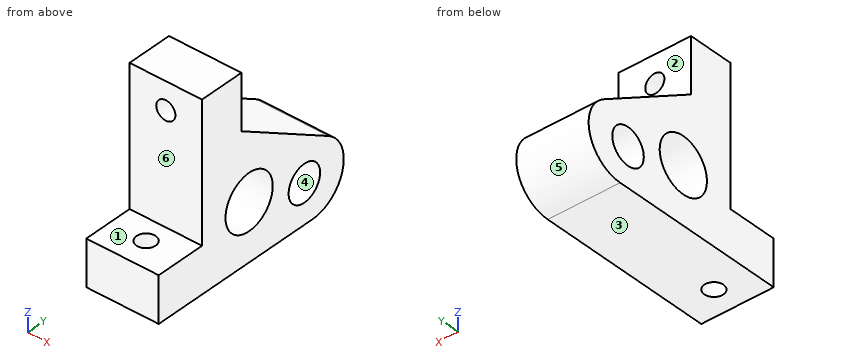
```python
from build123d import *

# Parameters (mm, degrees)
RESSALTO_EXTRUS_O1_DEPTH                       = 7.94
BROCA_DE_ROSQUEAR_PARA_TARRAXA_DE_M5X0_8_D     = 4.2
BROCA_DE_ROSQUEAR_PARA_TARRAXA_DE_M5X0_8_DEPTH = 20
BROCA_DE_ROSQUEAR_PARA_TARRAXA_DE_M5X0_8_TIP   = 1.2618073
BROCA_DE_ROSQUEAR_PARA_TARRAXA_DE_M5_2_D       = 4.2
BROCA_DE_ROSQUEAR_PARA_TARRAXA_DE_M5_2_DEPTH   = 20
BROCA_DE_ROSQUEAR_PARA_TARRAXA_DE_M5_2_TIP     = 1.2618073
BROCA_DE_ROSQUEAR_PARA_TARRAXA_DE_M5_3_D       = 4.2
BROCA_DE_ROSQUEAR_PARA_TARRAXA_DE_M5_3_DEPTH   = 20
BROCA_DE_ROSQUEAR_PARA_TARRAXA_DE_M5_3_TIP     = 1.2618073
BROCA_DE_ROSQUEAR_PARA_TARRAXA_DE_M5_4_D       = 4.2
BROCA_DE_ROSQUEAR_PARA_TARRAXA_DE_M5_4_DEPTH   = 20
BROCA_DE_ROSQUEAR_PARA_TARRAXA_DE_M5_4_TIP     = 1.2618073
ESBO_O10_R                                     = 6
ESBO_O10_R_2                                   = 4
CORTE_EXTRUS_O1_DEPTH                          = 57.108594707


with BuildPart() as part:
    # Esboço1 → Ressalto-extrusão1 (new, symmetric)
    with BuildSketch(Plane(origin=(0, 0, 0), x_dir=(0, 0, -1), z_dir=(1, 0, 0))):
        with BuildLine():
            Line((-40, 0), (-10, 0))
            Line((-10, 0), (-10, -11))
            Line((-10, -11), (0, -11))
            Line((0, -11), (0, 0))
            Line((0, 0), (0, 28))
            ThreePointArc((0, 28), (-5.881190502, 35.714314377), (-14.877661578, 32.086290643))
            Line((-14.877661578, 32.086290643), (-28, 10))
            Line((-28, 10), (-40, 10))
            Line((-40, 10), (-40, 0))
        make_face()
    extrude(amount=RESSALTO_EXTRUS_O1_DEPTH, both=True)

    # Broca de rosquear para tarraxa de M5x0.8
    with Locations(Plane(origin=(33.065, 10, -11.460196829), x_dir=(1, 0, 0), z_dir=(0, 1, 0))):
        with Locations((33.06, -45.460196829), (-33.065, -45.460196829)):
            Hole(BROCA_DE_ROSQUEAR_PARA_TARRAXA_DE_M5X0_8_D / 2, depth=BROCA_DE_ROSQUEAR_PARA_TARRAXA_DE_M5X0_8_DEPTH)
            with Locations((0, 0, -(BROCA_DE_ROSQUEAR_PARA_TARRAXA_DE_M5X0_8_DEPTH + BROCA_DE_ROSQUEAR_PARA_TARRAXA_DE_M5X0_8_TIP / 2))):  # 118° drill point
                Cone(0, BROCA_DE_ROSQUEAR_PARA_TARRAXA_DE_M5X0_8_D / 2, BROCA_DE_ROSQUEAR_PARA_TARRAXA_DE_M5X0_8_TIP, mode=Mode.SUBTRACT)

    # Broca de rosquear para tarraxa de M5 2
    with Locations(Plane(origin=(-33.06, 10, -11.460196829), x_dir=(1, 0, 0), z_dir=(0, 1, 0))):
        with Locations((33.06, -45.460196829), (-33.065, -45.460196829)):
            Hole(BROCA_DE_ROSQUEAR_PARA_TARRAXA_DE_M5_2_D / 2, depth=BROCA_DE_ROSQUEAR_PARA_TARRAXA_DE_M5_2_DEPTH)
            with Locations((0, 0, -(BROCA_DE_ROSQUEAR_PARA_TARRAXA_DE_M5_2_DEPTH + BROCA_DE_ROSQUEAR_PARA_TARRAXA_DE_M5_2_TIP / 2))):  # 118° drill point
                Cone(0, BROCA_DE_ROSQUEAR_PARA_TARRAXA_DE_M5_2_D / 2, BROCA_DE_ROSQUEAR_PARA_TARRAXA_DE_M5_2_TIP, mode=Mode.SUBTRACT)

    # Broca de rosquear para tarraxa de M5 3
    with Locations(Plane(origin=(33.065, -48.751665499, 0), x_dir=(-1, 0, 0), z_dir=(0, 0, -1))):
        with Locations((-33.06, 43.751665499), (33.065, 43.751665499)):
            Hole(BROCA_DE_ROSQUEAR_PARA_TARRAXA_DE_M5_3_D / 2, depth=BROCA_DE_ROSQUEAR_PARA_TARRAXA_DE_M5_3_DEPTH)
            with Locations((0, 0, -(BROCA_DE_ROSQUEAR_PARA_TARRAXA_DE_M5_3_DEPTH + BROCA_DE_ROSQUEAR_PARA_TARRAXA_DE_M5_3_TIP / 2))):  # 118° drill point
                Cone(0, BROCA_DE_ROSQUEAR_PARA_TARRAXA_DE_M5_3_D / 2, BROCA_DE_ROSQUEAR_PARA_TARRAXA_DE_M5_3_TIP, mode=Mode.SUBTRACT)

    # Broca de rosquear para tarraxa de M5 4
    with Locations(Plane(origin=(-33.06, -48.751665499, 0), x_dir=(-1, 0, 0), z_dir=(0, 0, -1))):
        with Locations((-33.06, 43.751665499), (33.065, 43.751665499)):
            Hole(BROCA_DE_ROSQUEAR_PARA_TARRAXA_DE_M5_4_D / 2, depth=BROCA_DE_ROSQUEAR_PARA_TARRAXA_DE_M5_4_DEPTH)
            with Locations((0, 0, -(BROCA_DE_ROSQUEAR_PARA_TARRAXA_DE_M5_4_DEPTH + BROCA_DE_ROSQUEAR_PARA_TARRAXA_DE_M5_4_TIP / 2))):  # 118° drill point
                Cone(0, BROCA_DE_ROSQUEAR_PARA_TARRAXA_DE_M5_4_D / 2, BROCA_DE_ROSQUEAR_PARA_TARRAXA_DE_M5_4_TIP, mode=Mode.SUBTRACT)

    # Esboço10 → Corte-extrusão1 (cut, through all)
    with BuildSketch(Plane(origin=(7.94, 0, 0), x_dir=(0, 0, -1), z_dir=(1, 0, 0))):
        with Locations((-12.404989074, 11.961998196)):
            Circle(ESBO_O10_R)
        with Locations((-8.551110249, 25.993478071)):
            Circle(ESBO_O10_R_2)
    extrude(amount=-CORTE_EXTRUS_O1_DEPTH, mode=Mode.SUBTRACT)


solid = part.part
```
Source: CAD feature listing. Evaluate the final solid. Frame: model axes, mm. Face numbers are marked on the shaded views. A direction names the side the tool comes from. Round coordinates to 2 decimals unless told otherwise and drop trailing zeros. Loops run counter-clockwise (first coordinate to the right, second up) from the corner with the lowest first, then second, coordinate; pieces in that order, holes last. Notation, with made-up numbers: M 25,-3.75 L 45,-3.75 A17 ccw 45,16.25 Z; hole C 3,74 d6. An arc over 180 degrees is marked long. Use a Markdown table: item, result. Add a question column.
1. Ray query, line 1 along X through (y, z) = (6.5, 34); line 2 along Y through (x, z) = (0, 7.5); line 3 along Z through (x, y) = (2, -1). Return the intervals inside material, ascending. Write a range as [from, to].
2. Contact query for flat-ended pins moving along their axis: pin 1 (9.5 mm diameter, centred on x = 2, z = 34, fed in from +Y); pin 2 (15.5 mm diameter, centred on y = 11.96, z = 12.4, fed in from -X); pin 3 (6.5 mm diameter, centred on x = 0, y = -5, fed in from +Z); pin 4 (5 mm diameter, centred on x = -0.5, z = 21.5, fed in from -Y). Output: stop coordinate, or through.
3. Cut plane D-D, the plane x = 0. Output: boundary loops of the cut face in (y, z), and give its area (3 significant figures).
4. Cut plane A-A, the plane y = 7. Output: boundary loops of the cut face in (x, z).
5. Cut plane B-B, the plane z = 34. Output: boundary loops of the cut face in (x, y), and give its area (3 significant figures).
6. Set-up query: the marked faces 1, 2 and 3. Return all of +Z, -Z, +X, -X, +Y, -Y with unobstructed straight access to the full face (end or side cutting, diameter ignored); none if empty.
7. Pull-direction query (Z, two-part tool) for the marked faces 4, 5 and 6; classes: +Z half, -Z half, draft (parallel to the pull), parting line (faces both ways), or undercut.
Solution:
| question | item | result |
|---|---|---|
| 1 | line 1 | x = [-7.94, -2.1], [2.1, 7.94] |
| 1 | line 2 | y = [-11, -7.1], [-2.9, 8.51], [15.42, 22.13], [29.85, 35.98] |
| 1 | line 3 | z = [0, 10] |
| 2 | pin 1 | stops at y = 10 |
| 2 | pin 2 | stops at x = -7.94 |
| 2 | pin 3 | stops at z = 10 |
| 2 | pin 4 | stops at y = 0 |
| 3 | outline | M -11,0 L -7.1,0 L -7.1,10 L -11,10 Z; M -2.9,0 L 28,0 A8 ccw 32.09,14.88 L 10,28 L 10,31.9 L 0,31.9 L 0,10 L -2.9,10 Z; M 0,36.1 L 10,36.1 L 10,40 L 0,40 Z; hole C 11.96,12.4 d12; hole C 25.99,8.55 d8 |
| 3 | area | 773 mm2 |
| 4 | outline | M -7.94,0 L 7.94,0 L 7.94,9.03 L -7.94,9.03 Z; M -7.94,15.78 L 7.94,15.78 L 7.94,40 L -7.94,40 Z; hole C 0,34 d4.2 |
| 5 | outline | M -7.94,0 L -2.1,0 L -2.1,10 L -7.94,10 Z; M 2.1,0 L 7.94,0 L 7.94,10 L 2.1,10 Z |
| 5 | area | 117 mm2 |
| 6 | face 1 | +Z, +X, -X, -Y |
| 6 | face 2 | +Z, +X, -X, +Y |
| 6 | face 3 | -Z, +X, -X, +Y, -Y |
| 7 | face 4 | undercut |
| 7 | face 5 | parting line |
| 7 | face 6 | draft |
